The model under review builds one solid part; all positions refer to its coordinate system, in mm. Round coordinates to 2 decimals unless told otherwise and drop trailing zeros. Loops run counter-clockwise (first coordinate to the right, second up) from the corner with the lowest first, then second, coordinate; pieces in that order, holes last. Notation, with made-up numbers: M 2,75 L 39,75 A20 cw 39,101 Z; hole C -25,26 d4. An arc over 180 degrees is marked long. Return JSON: item names as keys, results as strings. Group by question number.
Q1. Consider section C-C (x = 7). State the section outline as (y, z) points, and give its area (3 significant figures).
Q2. To check wall thickness, follow line 1 along Z through (x, y) = (-0.5, -2.1); line 2 along X through (y, z) = (-0.5, 70.5); line 3 along Z through (x, y) = (-4, -1.35). State the ranges of each line that lie inside material, in increasing order.
Q3. Consider section B-B (z = 98). State the section outline as (x, y) points, and give its area (3 significant figures).
Q4. Clearance check with a flat-ended pin moving along its axis: pin 1 Ø1.5 at (x, y) = (27, -1.5) entering from +Z. State where the tip first meets the part, or that it passes through.
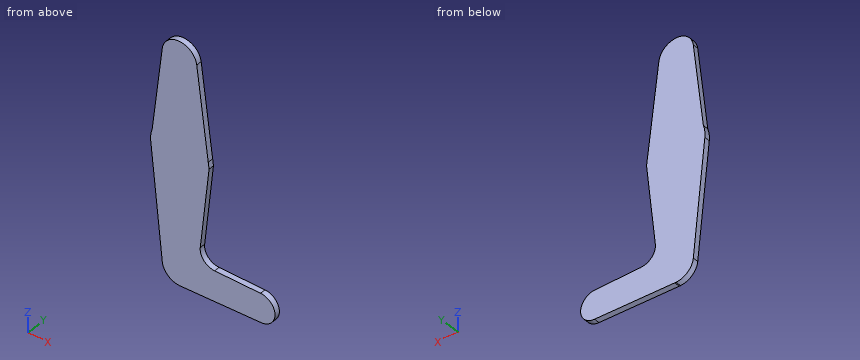
from build123d import *

# Parameters (mm, degrees)
F1_DEPTH = 3.048


with BuildPart() as f1:
    # F0 (on Front) → F1 (new body)
    with BuildSketch(Plane.XZ):
        with BuildLine():
            Line((9.525, 0), (0, 0))
            Line((0, 0), (0, 9.525))
            ThreePointArc((0, 9.525), (-7.063929059, 6.3895642457), (-9.4772553384, -0.9525))
            ThreePointArc((-9.4772553384, -0.9525), (-6.3895642457, -7.063929059), (0, -9.525))
            Line((0, -9.525), (0.6773435479, -9.500885786))
            ThreePointArc((0.6773435479, -9.500885786), (6.9705567315, -6.4912990883), (9.525, 0))
        make_face()
        with BuildLine():
            ThreePointArc((-9.4772553384, -0.9525), (-7.063929059, 6.3895642457), (0, 9.525))
            Line((0, 9.525), (0, 47.625))
            ThreePointArc((0, 47.625), (-10.6492737428, 51.7267849017), (-15.7954255641, 61.9125))
            Line((-15.7954255641, 61.9125), (-9.4772553384, -0.9525))
        make_face()
        with BuildLine():
            Line((0, 47.625), (0, 9.525))
            ThreePointArc((0, 9.525), (6.7351920908, 6.7351920908), (9.525, 0))
            Line((9.525, 0), (36.5125, 0))
            ThreePointArc((36.5125, 0), (38.8373399243, 5.6126600757), (44.45, 7.9375))
            Line((44.45, 7.9375), (19.2739472197, 7.9375))
            ThreePointArc((19.2739472197, 7.9375), (13.3609598068, 10.5733552714), (11.3688244585, 16.7331076944))
            Line((11.3688244585, 16.7331076944), (16.2005022244, 61.9125))
            Line((16.2005022244, 61.9125), (15.7504882915, 65.4843748585))
            ThreePointArc((15.7504882915, 65.4843748585), (15.8438414948, 64.4941386655), (15.875, 63.5))
            ThreePointArc((15.875, 63.5), (11.2253201513, 52.2746798487), (0, 47.625))
        make_face()
        with BuildLine():
            Line((36.5125, 0), (9.525, 0))
            ThreePointArc((9.525, 0), (6.9705567315, -6.4912990883), (0.6773435479, -9.500885786))
            Line((0.6773435479, -9.500885786), (44.7324052746, -7.9324746146))
            ThreePointArc((44.7324052746, -7.9324746146), (38.9380895153, -5.7116327839), (36.5125, 0))
        make_face()
        with BuildLine():
            ThreePointArc((-15.7954255641, 61.9125), (-10.6492737428, 51.7267849017), (0, 47.625))
            Line((0, 47.625), (0, 79.375))
            ThreePointArc((0, 79.375), (-9.1908363712, 76.4438847259), (-14.9877324754, 68.7329246359))
            Line((-14.9877324754, 68.7329246359), (-15.7954255641, 61.9125))
        make_face()
        with BuildLine():
            Line((0, 79.375), (0, 47.625))
            ThreePointArc((0, 47.625), (11.2253201513, 52.2746798487), (15.875, 63.5))
            ThreePointArc((15.875, 63.5), (15.8438414948, 64.4941386655), (15.7504882915, 65.4843748585))
            ThreePointArc((15.7504882915, 65.4843748585), (10.5003255693, 75.4062499528), (0, 79.375))
        make_face()
        with BuildLine():
            ThreePointArc((44.45, 7.9375), (38.8373399243, 5.6126600757), (36.5125, 0))
            ThreePointArc((36.5125, 0), (38.9380895153, -5.7116327839), (44.7324052746, -7.9324746146))
            ThreePointArc((44.7324052746, -7.9324746146), (50.1616327839, -5.5119104847), (52.3875, 0))
            ThreePointArc((52.3875, 0), (50.0626600757, 5.6126600757), (44.45, 7.9375))
        make_face()
        with BuildLine():
            ThreePointArc((0, -9.525), (0.3388863295, -9.5189695375), (0.6773435479, -9.500885786))
            Line((0.6773435479, -9.500885786), (0, -9.525))
        make_face()
        with BuildLine():
            ThreePointArc((-14.9877324754, 68.7329246359), (-9.1908363712, 76.4438847259), (0, 79.375))
            Line((0, 79.375), (0, 104.775))
            ThreePointArc((0, 104.775), (-7.1202192788, 107.9732233782), (-9.4589053806, 115.4201490977))
            Line((-9.4589053806, 115.4201490977), (-14.9877324754, 68.7329246359))
        make_face()
        with BuildLine():
            Line((0, 104.775), (0, 79.375))
            ThreePointArc((0, 79.375), (10.5003255693, 75.4062499528), (15.7504882915, 65.4843748585))
            Line((15.7504882915, 65.4843748585), (9.4502929642, 115.490625))
            ThreePointArc((9.4502929642, 115.490625), (9.5063048942, 114.896483242), (9.525, 114.3))
            ThreePointArc((9.525, 114.3), (6.7351920908, 107.5648079092), (0, 104.775))
        make_face()
        with BuildLine():
            ThreePointArc((-14.9877324754, 68.7329246359), (-15.764842301, 65.3669151629), (-15.7954255641, 61.9125))
            Line((-15.7954255641, 61.9125), (-14.9877324754, 68.7329246359))
        make_face()
        with BuildLine():
            ThreePointArc((-9.4589053806, 115.4201490977), (-7.1202192788, 107.9732233782), (0, 104.775))
            ThreePointArc((0, 104.775), (6.7351920908, 107.5648079092), (9.525, 114.3))
            ThreePointArc((9.525, 114.3), (9.5063048942, 114.896483242), (9.4502929642, 115.490625))
            ThreePointArc((9.4502929642, 115.490625), (-0.0355000934, 123.8249338446), (-9.4589053806, 115.4201490977))
        make_face()
        with BuildLine():
            Line((0, 9.525), (0, 0))
            Line((0, 0), (9.525, 0))
            ThreePointArc((9.525, 0), (6.7351920908, 6.7351920908), (0, 9.525))
        make_face()
    extrude(amount=F1_DEPTH)


solid = f1.part
Values:
{
 "1": {"outline": "M -3.05,-9.28 L 0,-9.28 L 0,120.76 L -3.05,120.76 Z", "area": "396 mm2"},
 "2": {"line 1": "z = -9.51 to 123.81", "line 2": "x = -14.78 to 15.12", "line 3": "z = -8.64 to 122.94"},
 "3": {"outline": "M -11.52,-3.05 L 11.65,-3.05 L 11.65,0 L -11.52,0 Z", "area": "70.6 mm2"},
 "4": {"pin 1": "stops at z = 7.94"}
}
